Source: CAD feature listing. Evaluate the final solid. Frame: model axes, mm. Round coordinates to 2 decimals unless told otherwise and drop trailing zeros. Write each loop counter-clockwise with the first axis right and the second up, starting at its lowest first coordinate (ties: lowest second). Pieces come first, ordered by that corner, then holes.
from build123d import *

# Parameters (mm, degrees)
PAD_DEPTH         = 2
POCKET_DEPTH      = 25
POCKET_DEPTH_BACK = -25
FILLET_R          = 0.99


with BuildPart() as part:
    # Sketch → Pad (new body)
    with BuildSketch(Plane.XY):
        Polygon((0, -25), (22.318456, -11.264392), (22.318456, 11.264392), (0, 25), align=None)
    extrude(amount=PAD_DEPTH)

    # Sketch001 → Pocket (cut, two sides)
    with BuildSketch(Plane.XZ) as pocket_sk:
        Polygon((0, 2), (0.57735, 1), (0, 0), (-0.786644, 0.221257), (-0.914664, 1.821517), align=None)
    extrude(amount=-POCKET_DEPTH, mode=Mode.SUBTRACT)
    extrude(pocket_sk.sketch, amount=-POCKET_DEPTH_BACK, mode=Mode.SUBTRACT)

    # Fillet
    fillet_edges = [part.edges().sort_by_distance(p)[0] for p in [
        (11.159228, 18.132196, 0),
        (11.159228, 18.132196, 2),
        (22.318456, 0, 0),
        (11.159228, -18.132196, 0),
        (22.318456, 0, 2),
        (11.159228, -18.132196, 2),
    ]]
    fillet(fillet_edges, radius=FILLET_R)


solid = part.part
1) Pull-direction query (Z, two-part tool) for faces 1 (the face through (22.02, 0.16, 1.72)), 2 (the face through (0.285, 0.346, 1.507)), 3 (the face through (22.04, 0.16, 0.3)), 4 (the face through (0.293, 0.346, 0.507)); classes: released by +Z, released by -Z, zero draft, split by the parting line, or undercut.
Taken from the geometry:
face 1: released by +Z
face 2: undercut
face 3: released by -Z
face 4: undercut
2) Material intervals for line 1 (Y direction, x = 17.25, z = 1.75); line 2 (X direction, y = -12.5, z = 1.6); line 3 (X direction, y = -1, z = 1.35), sorted ascending.
Taken from the geometry:
line 1: y = -13.99 to 13.99
line 2: x = 0.23 to 19.94
line 3: x = 0.38 to 22.26
3) Section query B-B on z = 0.55. Return the cut outline in (x, y), then the cut area to 3 significant figures.
Taken from the geometry:
outline: (0.32, -24.68) - (22.22, -11.21) - (22.22, 11.21) - (0.32, 24.68) - close
area: 786 mm2
